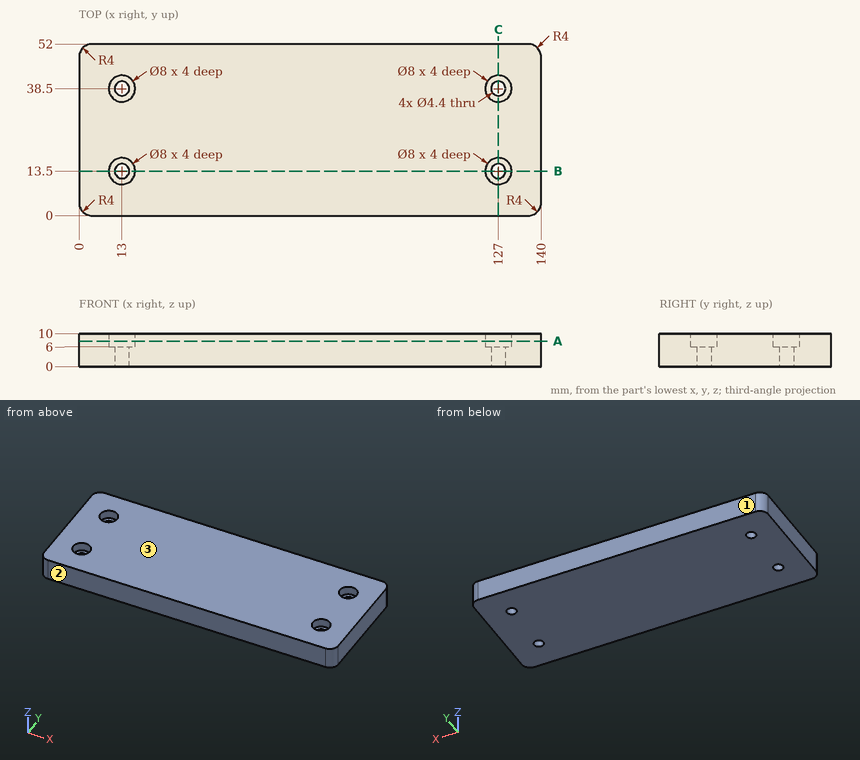
Print and shaded views of the part. All mm, measured from the part's lowest x, y and z. Give positions to 0.01 mm unless a question says otherwise; leave off trailing zeros. Write each loop counter-clockwise with the first axis right and the second up, starting at its lowest first coordinate (ties: lowest second). Pieces come first, ordered by that corner, then holes. Notation, with made-up numbers: (89.5, -3) -> (126.5, -3) arc R23 cw to (126.5, 29) -> close; hole circle Ø8 at (47, 66). An arc over 180 degrees is marked (long way). Use CSV: the item, a comma, the result in double quotes. Start each with the question number.
1) Pin check, flat tip, straight feed: P1, Ø5, axis at x = 13, y = 38.5, coming from the +Z side. Stop position of the tip, or through.
2) Cut at A-A on z = 7.75. List the corners of the cut face in (x, y).
3) Two-plate mould, pull along Y, no slides. Class the marked faces 1, 2 and 3: released by +Y, released by -Y, zero draft, split by the parting line, or undercut.
4) Cut at B-B on y = 13.5. List the corners of the cut face in (x, z).
5) Cut at C-C on x = 127. List the corners of the cut face in (y, z).
6) Drill centre lines: L1, parallel to Y at x = 127, z = 7.15; L2, parallel to X at y = 38.5, z = 9.2; L3, parallel to Y at x = 127, z = 1.9. Where is each one in solid material? Low to high.
Final values:
1,P1,"stops at z = 6"
2,outline,"(0, 4) arc R4 ccw to (4, 0) -> (136, 0) arc R4 ccw to (140, 4) -> (140, 48) arc R4 ccw to (136, 52) -> (4, 52) arc R4 ccw to (0, 48) -> close; hole circle Ø8 at (13, 13.5); hole circle Ø8 at (13, 38.5); hole circle Ø8 at (127, 13.5); hole circle Ø8 at (127, 38.5)"
3,face 1,"released by +Y"
3,face 2,"released by -Y"
3,face 3,"zero draft"
4,outline,"(0, 0) -> (10.8, 0) -> (10.8, 6) -> (9, 6) -> (9, 10) -> (0, 10) -> close; (15.2, 0) -> (124.8, 0) -> (124.8, 6) -> (123, 6) -> (123, 10) -> (17, 10) -> (17, 6) -> (15.2, 6) -> close; (129.2, 0) -> (140, 0) -> (140, 10) -> (131, 10) -> (131, 6) -> (129.2, 6) -> close"
5,outline,"(0, 0) -> (11.3, 0) -> (11.3, 6) -> (9.5, 6) -> (9.5, 10) -> (0, 10) -> close; (15.7, 0) -> (36.3, 0) -> (36.3, 6) -> (34.5, 6) -> (34.5, 10) -> (17.5, 10) -> (17.5, 6) -> (15.7, 6) -> close; (40.7, 0) -> (52, 0) -> (52, 10) -> (42.5, 10) -> (42.5, 6) -> (40.7, 6) -> close"
6,L1,"y = 0 to 9.5, 17.5 to 34.5, 42.5 to 52"
6,L2,"x = 0 to 9, 17 to 123, 131 to 140"
6,L3,"y = 0 to 11.3, 15.7 to 36.3, 40.7 to 52"
